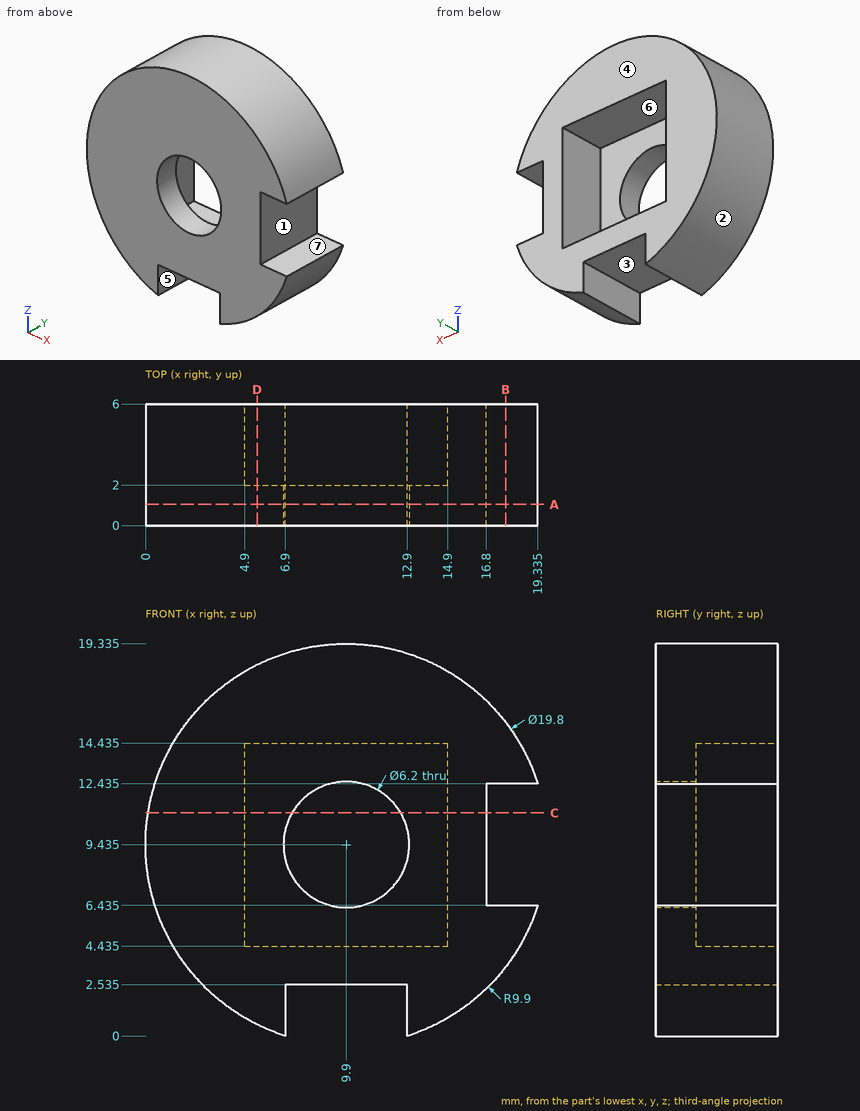
Verification items for this drawing (mm, ordinates from the low corner). A direction names the side the tool comes from. Give positions to 0.01 mm unless a question says otherwise; leave off trailing zeros. Write each loop counter-clockwise with the first axis right and the second up, starting at its lowest first coordinate (ties: lowest second). Pieces come first, ordered by that corner, then holes. Notation, with made-up numbers: (70.25, 14.5) -> (88.25, 14.5) arc R28 cw to (88.25, 34.5) -> close; hole circle Ø1 at (48, -18.75). An arc over 180 degrees is marked (long way). Use one line per item in the form item = value.
Item 1: Sectioned sample at A-A on y = 1.05. Enter the section's corners in (x, z) (1 decimal).
Results list:
outline = (6.9, 0) -> (6.9, 2.5) -> (12.9, 2.5) -> (12.9, 0) arc R9.9 ccw to (19.3, 6.4) -> (16.8, 6.4) -> (16.8, 12.4) -> (19.3, 12.4) arc R9.9 ccw (long way) to start; hole circle Ø6.2 at (9.9, 9.4)
Item 2: Depth check by flat-ended pin: pin 1 Ø1.8 at (x, y) = (8.5, 2.5) entering from -Z (1 decimal); pin 2 Ø3 at (x, y) = (3, 4.5) entering from +Z; pin 3 Ø1.3 at (y, z) = (1.5, 0.5) entering from -X. Enter the tip coordinate at first touch or a pass-through.
Results list:
pin_1 = 2.5
pin_2 = 17.73
pin_3 = 4.48
Item 3: Mould release check, pull along X, two halves, no side actions. Record for the marked faces 1, 2, 3 and 4: released by +X, released by -X, zero draft, split by the parting line, or undercut.
Results list:
face_1 = released by +X
face_2 = split by the parting line
face_3 = undercut
face_4 = zero draft
Item 4: Sectioned sample at D-D on x = 5.5. Enter the section's corners in (y, z) (1 decimal).
Results list:
outline = (0, 0.6) -> (6, 0.6) -> (6, 4.4) -> (2, 4.4) -> (2, 14.4) -> (6, 14.4) -> (6, 18.3) -> (0, 18.3) -> close
Item 5: Scan lines: line 1 (Y direction, x = 6, z = 5.25); line 2 (X direction, y = 0.35, z = 10.25) (1 decimal); line 3 (X direction, y = 2.25, z = 7.25) (1 decimal). Record each from-to range of solid material in increasing order.
Results list:
line_1 = 0 to 2
line_2 = 0 to 6.9, 12.9 to 16.8
line_3 = 0.2 to 4.9, 14.9 to 16.8
Item 6: Access from +Z, -Z, +X, -X, +Y, -Y to the whole of each face (thin tool, end or side, straight path). Record for the marked faces 5, 6 and 7.
Results list:
face_5 = -Z, +Y, -Y
face_6 = +Y
face_7 = +X, +Y, -Y
Item 7: Sectioned sample at C-C on z = 11. Enter the section's corners in (x, y) (1 decimal).
Results list:
outline = (0.1, 0) -> (7.2, 0) -> (7.2, 2) -> (4.9, 2) -> (4.9, 6) -> (0.1, 6) -> close; (12.6, 0) -> (16.8, 0) -> (16.8, 6) -> (14.9, 6) -> (14.9, 2) -> (12.6, 2) -> close
Item 8: Sectioned sample at B-B on x = 17.75. Enter the section's corners in (y, z) (1 decimal).
Results list:
outline = (0, 3.4) -> (6, 3.4) -> (6, 6.4) -> (0, 6.4) -> close; (0, 12.4) -> (6, 12.4) -> (6, 15.5) -> (0, 15.5) -> close
